Input: dimensioned drawing with shaded views. Units: mm. Origin: part minimum x, y, z. A direction names the side the tool comes from. Round coordinates to 2 decimals unless told otherwise and drop trailing zeros. Write each loop counter-clockwise with the first axis right and the second up, starting at its lowest first coordinate (ties: lowest second). Pieces come first, ordered by that corner, then holes. Notation, with made-up numbers: (-1, 64.5) -> (5, 64.5) arc R29 cw to (5, 92.5) -> close; hole circle Ø3 at (48.25, -13). An arc over 180 degrees is marked (long way). One line per item, written item: value. Start each with the question number.
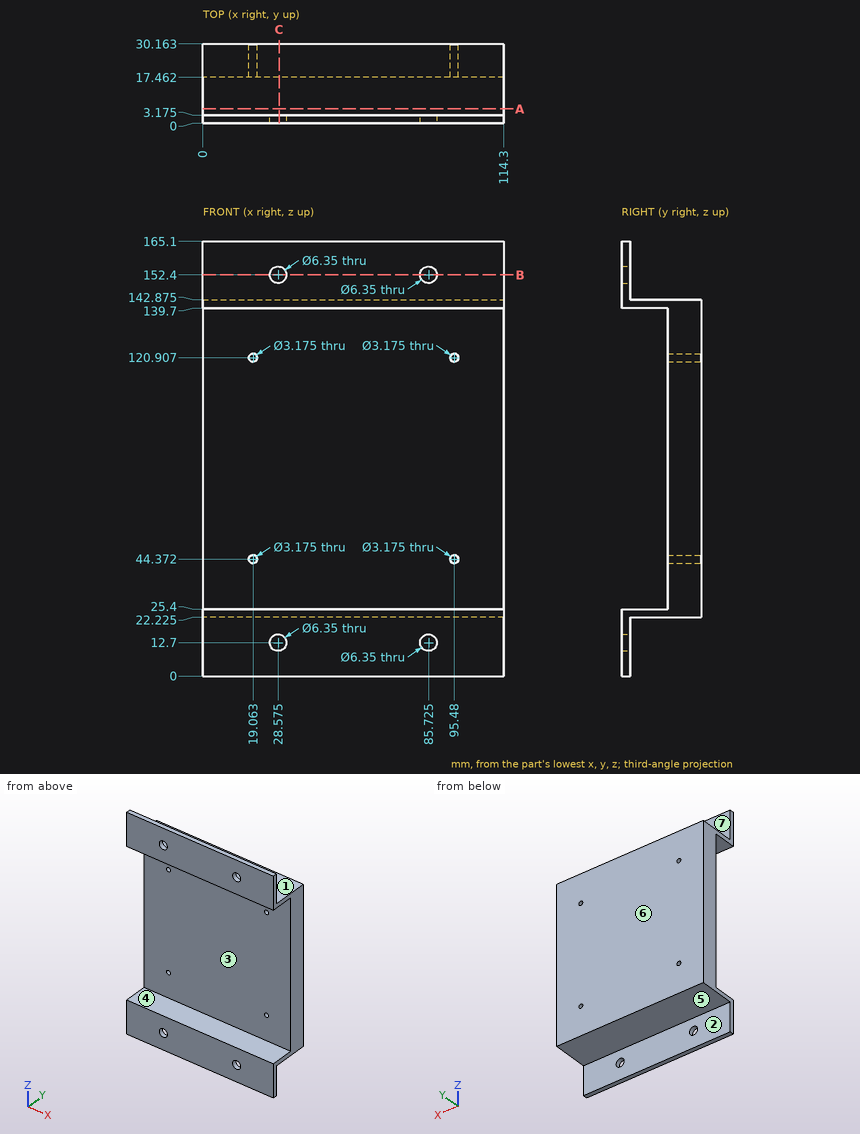
(1) Set-up query: the marked faces 4, 5, 6 and 7. Return all of +Z, -Z, +X, -X, +Y, -Y with unobstructed straight access to the full face (end or side cutting, diameter ignored); none if empty.
(2) Pull-direction query (Z, two-part tool) for the marked faces 1, 2 and 3; classes: pulls with the +Z half, pulls with the -Z half, needs draft (parallel to the pull), parting line crosses it, or undercut.
(3) Section query C-C (x = 29). Output: boundary loops of the cut face in (y, z) (1 decimal), and give its area (3 significant figures).
(4) Pin query (flat end, axial travel): pin 1 (12 mm diameter, centred on x = 91, y = 8, fed in from -Z); pin 2 (8.5 mm diameter, centred on x = 57, y = 12.5, fed in from -Z) (1 decimal); pin 3 (3 mm diameter, centred on x = 19.06, z = 44.37, fed in from -Y); pin 4 (18 mm diameter, centred on x = 80.5, z = 10, fed in from +Y) (1 decimal). Return the tip coordinate at first contact, or that it passes through.
(5) Section query B-B (z = 152.4). Count the separate pieces of the cut face and the enclosed holes in it.
(6) Line query: probe 1 along Z at (x, y) = (85.5, 6.5) (1 decimal); probe 2 along Z at (x, y) = (18, 2.5); probe 3 along X at (y, z) = (1, 12). Output: solid intervals per line, ascending.
(7) Section query A-A (y = 5.5). Output: boundary loops of the cut face in (x, z) (1 decimal).
Results list:
1. face 4: +X, -X, -Y
1. face 5: -Z, +X, -X, +Y
1. face 6: +Z, -Z, +X, -X, +Y
1. face 7: +Z, +X, -X, +Y
2. face 1: pulls with the +Z half
2. face 2: needs draft
2. face 3: undercut
3. outline: (0, 0) -> (3.2, 0) -> (3.2, 9.6) -> (0, 9.6) -> close; (0, 15.8) -> (3.2, 15.8) -> (3.2, 22.2) -> (30.2, 22.2) -> (30.2, 142.9) -> (3.2, 142.9) -> (3.2, 149.3) -> (0, 149.3) -> (0, 139.7) -> (17.5, 139.7) -> (17.5, 25.4) -> (0, 25.4) -> close; (0, 155.5) -> (3.2, 155.5) -> (3.2, 165.1) -> (0, 165.1) -> close
3. area: 1,740 mm^2
4. pin 1: stops at z = 0
4. pin 2: stops at z = 22.2
4. pin 3: passes through
4. pin 4: stops at y = 3.2
5. separate pieces: 3
5. enclosed holes: 0
6. probe 1: z = 22.2 to 25.4, 139.7 to 142.9
6. probe 2: z = 0 to 25.4, 139.7 to 165.1
6. probe 3: x = 0 to 25.48, 31.67 to 82.63, 88.82 to 114.3
7. outline: (0, 22.2) -> (114.3, 22.2) -> (114.3, 25.4) -> (0, 25.4) -> close; (0, 139.7) -> (114.3, 139.7) -> (114.3, 142.9) -> (0, 142.9) -> close
